Here's how the part is built. I have some questions about the finished solid (model axes, mm). Face numbers are marked on the shaded views. A direction names the side the tool comes from. Give positions to 0.01 mm unless a question says otherwise; leave off trailing zeros. Write each loop counter-clockwise with the first axis right and the second up, starting at its lowest first coordinate (ties: lowest second). Pieces come first, ordered by that corner, then holes. Notation, with made-up numbers: (44.25, 27) - (78.25, 27) arc R12 ccw to (78.25, 44) - close; hole circle Ø5 at (37, 69.25). An arc over 180 degrees is marked (long way). Use one line per item in the form item = value. Start each with the question number.
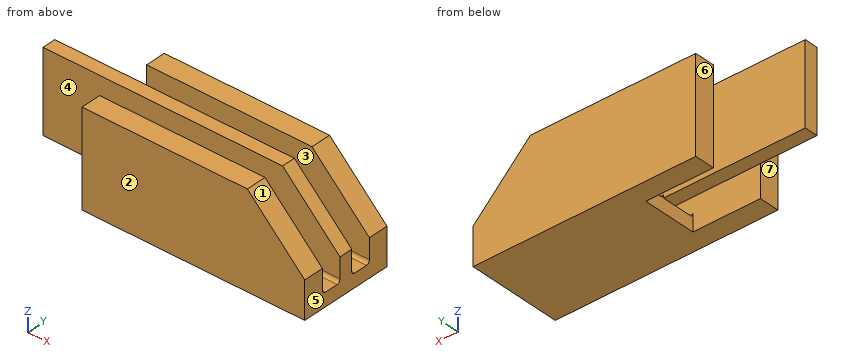
from build123d import *

# Parameters (mm, degrees)
F0_W     = 292.1
F0_H     = 44.45
F1_DEPTH = 25.4
F3_DEPTH = 152.4
F4_W     = 292.1
F4_H     = 38.1
F5_DEPTH = 152.4
F6_SIZE  = 107.95
F7_W     = 25.4
F7_H     = 152.4
F8_DEPTH = 266.7
F9_R     = 6.35
F10_R    = 6.35


with BuildPart() as f1:
    # F0 (on Top) → F1 (new body)
    with BuildSketch(Plane.XY):
        Polygon((390.6061206371, 24.8817224056), (-28.4938793629, 24.8817224056), (-28.4938793629, -13.2182775944), (98.5061206371, -13.2182775944), (390.6061206371, -13.2182775944), align=None)
        with Locations((244.5561206371, -35.4432775944)):
            Rectangle(F0_W, F0_H)
        Polygon((390.6061206371, -70.3682775944), (390.6061206371, -57.6682775944), (98.5061206371, -57.6682775944), (98.5061206371, -64.0182775944), (98.5061206371, -70.3682775944), align=None)
        with Locations((244.5561206371, -92.5932775944)):
            Rectangle(F0_W, F0_H)
        Polygon((390.6061206371, -152.9182775944), (390.6061206371, -114.8182775944), (98.5061206371, -114.8182775944), (-28.4938793629, -114.8182775944), (-28.4938793629, -152.9182775944), align=None)
    extrude(amount=F1_DEPTH)

    # F3 (add): a face of the model
    f3_faces = [f1.faces().sort_by_distance(p)[0] for p in [
        (211.6425080716, -64.0182775944, 25.4),
    ]]
    extrude(f3_faces, amount=F3_DEPTH)

    # F4 (on face) → F5 (cut)
    with BuildSketch(Plane.XY.offset(177.8)):
        with Locations((244.5561206371, -32.2682775944)):
            Rectangle(F4_W, F4_H)
        with Locations((244.5561206371, -95.7682775944)):
            Rectangle(F4_W, F4_H)
    extrude(amount=-F5_DEPTH, mode=Mode.SUBTRACT)

    # F6
    f6_edges = [f1.edges().sort_by_distance(p)[0] for p in [
        (390.606121, -133.868278, 177.8),
        (390.606121, -64.018278, 177.8),
        (390.606121, 5.831722, 177.8),
    ]]
    chamfer(f6_edges, length=F6_SIZE)

    # F7 (on face) → F8 (join)
    with BuildSketch(Plane(origin=(98.5061206371, 0, 0), x_dir=(0, -1, 0), z_dir=(-1, 0, 0))):
        with Locations((64.0182775944, 101.6)):
            Rectangle(F7_W, F7_H)
    extrude(amount=F8_DEPTH)

    # F9
    f9_edges = [f1.edges().sort_by_distance(p)[0] for p in [
        (244.556121, -114.818278, 25.4),
    ]]
    fillet(f9_edges, radius=F9_R)

    # F10
    f10_edges = [f1.edges().sort_by_distance(p)[0] for p in [
        (244.556121, -51.318278, 25.4),
        (244.556121, -76.718278, 25.4),
        (244.556121, -13.218278, 25.4),
    ]]
    fillet(f10_edges, radius=F10_R)


solid = f1.part
1. I want a section at C-C, the plane x = 258.5. List the corners of the cut face in (y, z) for me, then the cut area to 3 significant figures.
2. For P1, Ø12, axis at y = -129, z = 125, coming from the -X side; P2, Ø12.5, axis at x = 272, y = -32.5, coming from the +Z side; P3, Ø12.5, axis at x = 18.5, y = -70, coming from the -Z side, each with a flat end and sliding along its axis, tell me the tip position at first contact or that it passes through.
3. I want a section at D-D, the plane y = 6. List the corners of the cut face in (x, z) for me, then the cut area to 3 significant figures.
4. I want a section at A-A, the plane x = -16. List the corners of the cut face in (y, z) for me.
5. Please list where these lines run through material, in increasing order: line 1 (Y direction, x = 30, z = 133.5); line 2 (Y direction, x = -91.5, z = 33); line 3 (Z direction, x = 259.5, y = -91).
6. I want a section at B-B, the plane z = 89. List the corners of the cut face in (x, y) for me.
7. For the marked faces 5, 6 and 7, which set-ups out of +Z, -Z, +X, -X, +Y, -Y let a thin tool reach every point of the face, with its end or its side?
8. We'd pull the mould along Y, two halves only. Please class the marked faces 1, 2, 3 and 4: pulls with the +Y half, pulls with the -Y half, needs draft (parallel to the pull), parting line crosses it, or undercut.
Result sheet:
q1.outline = (-152.92, 0) - (24.88, 0) - (24.88, 177.8) - (-13.22, 177.8) - (-13.22, 31.75) arc R6.35 cw to (-19.57, 25.4) - (-44.97, 25.4) arc R6.35 cw to (-51.32, 31.75) - (-51.32, 177.8) - (-76.72, 177.8) - (-76.72, 31.75) arc R6.35 cw to (-83.07, 25.4) - (-108.47, 25.4) arc R6.35 cw to (-114.82, 31.75) - (-114.82, 177.8) - (-152.92, 177.8) - close
q1.area = 20,000 mm2
q2.P1 = -28.49
q2.P2 = 25.4
q2.P3 = 25.4
q3.outline = (-28.49, 0) - (390.61, 0) - (390.61, 69.85) - (282.66, 177.8) - (-28.49, 177.8) - close
q3.area = 68,700 mm2
q4.outline = (-152.92, 0) - (-114.82, 0) - (-114.82, 177.8) - (-152.92, 177.8) - close; (-76.72, 25.4) - (-51.32, 25.4) - (-51.32, 177.8) - (-76.72, 177.8) - close; (-13.22, 0) - (24.88, 0) - (24.88, 177.8) - (-13.22, 177.8) - close
q5.line_1 = -152.92 to -114.82, -76.72 to -51.32, -13.22 to 24.88
q5.line_2 = -76.72 to -51.32
q5.line_3 = 0 to 25.4
q6.outline = (-168.19, -76.72) - (371.46, -76.72) - (371.46, -51.32) - (-168.19, -51.32) - close; (-28.49, -152.92) - (371.46, -152.92) - (371.46, -114.82) - (-28.49, -114.82) - close; (-28.49, -13.22) - (371.46, -13.22) - (371.46, 24.88) - (-28.49, 24.88) - close
q7.face_5 = +Z, -Z, +X, +Y, -Y
q7.face_6 = +Z, -Z, -X, +Y
q7.face_7 = +Z, -Z, -X, -Y
q8.face_1 = needs draft
q8.face_2 = pulls with the -Y half
q8.face_3 = undercut
q8.face_4 = undercut
